Geometry check sheet. Reference: the model listing, model coordinates, mm. Round coordinates to 2 decimals unless told otherwise and drop trailing zeros. Loops run counter-clockwise (first coordinate to the right, second up) from the corner with the lowest first, then second, coordinate; pieces in that order, holes last. Notation, with made-up numbers: (-17.75, 70) -> (38.25, 70) arc R6 ccw to (38.25, 77) -> close; hole circle Ø5 at (51.5, 29). An arc over 180 degrees is marked (long way). Use one line per item in the form item = value.
from build123d import *
from OCP.BRepFilletAPI import BRepFilletAPI_MakeChamfer

# Parameters (mm, degrees)
SKETCH_1_W          = 33.5
SKETCH_1_H          = 32
SKETCH_1_R          = 1
SKETCH_1_W_2        = 23.5
SKETCH_1_H_2        = 24.25
EXTRUDE_1_DEPTH     = 2
SKETCH_2_W          = 12
SKETCH_2_H          = 12
SKETCH_2_R          = 4
EXTRUDE_2_DEPTH     = 2.2
EXTRUDE_3_DEPTH     = 12
EXTRUDE_4_DEPTH     = 12
SKETCH_5_W          = 33.5
SKETCH_5_H          = 2
EXTRUDE_5_DEPTH     = 14
SKETCH_7_W          = 2
SKETCH_7_H          = 32
EXTRUDE_6_DEPTH     = 16
SKETCH_9_R          = 3.625
CUT_EXTRUDE_1_DEPTH = 1
SKETCH_10_R         = 2.25
CUT_EXTRUDE_2_DEPTH = 1
EXTRUDE_START       = -2
SKETCH_11_R         = 5
SKETCH_11_R_2       = 3.625
EXTRUDE_7_DEPTH     = 2
FILLET_1_R          = 1
SKETCH_12_R         = 3
SKETCH_12_R_2       = 1.5
EXTRUDE_8_DEPTH     = 2
FILLET_2_R          = 1
CUT_EXTRUDE_START   = 2
SKETCH_13_R         = 1.5
CUT_EXTRUDE_3_DEPTH = 2
SKETCH_19_W         = 3.200973594
SKETCH_19_H         = 7
CUT_EXTRUDE_7_DEPTH = 10
CUT_EXTRUDE_8_DEPTH = 42
SKETCH_22_R         = 0.75
CUT_EXTRUDE_9_DEPTH = 5
CHAMFER_1_SIZE      = 1
CHAMFER_1_SIZE2     = 2


with BuildPart() as part:
    # Sketch 1 → Extrude 1 (new body)
    with BuildSketch(Plane.XY):
        with Locations((-5.75, -6.125)):
            Rectangle(SKETCH_1_W, SKETCH_1_H)
        with Locations((-20, 0)):
            Circle(SKETCH_1_R, mode=Mode.SUBTRACT)
        with Locations(Location((8.5, 0, 0), (0, 0, 180))):
            Circle(SKETCH_1_R, mode=Mode.SUBTRACT)
        with Locations(Location((-20, -12.25, 0), (0, 0, 180))):
            Circle(SKETCH_1_R, mode=Mode.SUBTRACT)
        with Locations((8.5, -12.25)):
            Circle(SKETCH_1_R, mode=Mode.SUBTRACT)
        with Locations((-5.75, -6.125)):
            Rectangle(SKETCH_1_W_2, SKETCH_1_H_2, mode=Mode.SUBTRACT)
    extrude(amount=EXTRUDE_1_DEPTH)



with BuildPart() as body_2:
    # Sketch 2 → Extrude 2 (new body)
    with BuildSketch(Plane.XY.offset(9)):
        with Locations((0, -12.25)):
            Rectangle(SKETCH_2_W, SKETCH_2_H)
        with Locations((0, -12.25)):
            Circle(SKETCH_2_R, mode=Mode.SUBTRACT)
    extrude(amount=-EXTRUDE_2_DEPTH)


with BuildPart() as part_1:
    add(part.part)

    add(body_2.part)  # Extrude 3 merges body 2
    # Sketch 3 → Extrude 3 (add)
    with BuildSketch(Plane.ZY.offset(6)):
        Polygon((9, -18.25), (2, -18.25), (2, -22.125), (9, -20.25), align=None)
    extrude(amount=-EXTRUDE_3_DEPTH)

    # Sketch 4 → Extrude 4 (add)
    with BuildSketch(Plane.ZY.offset(6)):
        Polygon((6.8, -6.25), (9, -6.25), (9, 9.5), (2, 9.5), (2, 6), (6.8, 6), align=None)
    extrude(amount=-EXTRUDE_4_DEPTH)

    # Sketch 5 → Extrude 5 (add)
    with BuildSketch(Plane(origin=(0, 0, 0), x_dir=(-1, 0, 0), z_dir=(0, 0, -1))):
        with Locations((5.75, 8.875)):
            Rectangle(SKETCH_5_W, SKETCH_5_H)
        with Locations((5.75, -21.125)):
            Rectangle(SKETCH_5_W, SKETCH_5_H)
    extrude(amount=EXTRUDE_5_DEPTH)

    # Sketch 7 → Extrude 6 (add)
    with BuildSketch(Plane.XY.offset(2)):
        with Locations((-23.5, -6.125)):
            Rectangle(SKETCH_7_W, SKETCH_7_H)
        with Locations((12, -6.125)):
            Rectangle(SKETCH_7_W, SKETCH_7_H)
    extrude(amount=-EXTRUDE_6_DEPTH)

    # Sketch 9 → Cut-Extrude 1 (cut)
    with BuildSketch(Plane(origin=(-24.5, 0, 0), x_dir=(0, 0, -1), z_dir=(1, 0, 0))):
        with Locations(Location((8, -12.25, 0), (0, 0, 90))):
            Circle(SKETCH_9_R)
    extrude(amount=CUT_EXTRUDE_1_DEPTH, mode=Mode.SUBTRACT)

    # Sketch 10 → Cut-Extrude 2 (cut)
    with BuildSketch(Plane.ZY.offset(23.5)):
        with Locations(Location((-8, -12.25, 0), (0, 0, 270))):
            Circle(SKETCH_10_R)
    extrude(amount=-CUT_EXTRUDE_2_DEPTH, mode=Mode.SUBTRACT)

    # Sketch 11 → Extrude 7 (add)
    with BuildSketch(Plane(origin=(-24.5, 0, 0), x_dir=(0, 0, -1), z_dir=(1, 0, 0)).offset(EXTRUDE_START)):
        with Locations(Location((8, -12.25, 0), (0, 0, 90))):
            Circle(SKETCH_11_R)
        with Locations(Location((8, -12.25, 0), (0, 0, 90))):
            Circle(SKETCH_11_R_2, mode=Mode.SUBTRACT)
    extrude(amount=EXTRUDE_7_DEPTH)

    # Fillet 1
    fillet_1_edges = [part_1.edges().sort_by_distance(p)[0] for p in [
        (-24.5, -17.25, -8),
    ]]
    fillet(fillet_1_edges, radius=FILLET_1_R - 0.0001)  # a hair under: the kernel refuses the full size

    # Sketch 12 → Extrude 8 (add)
    with BuildSketch(Plane.ZY.offset(-13)):
        with Locations(Location((-8, -12.25, 0), (0, 0, 270))):
            Circle(SKETCH_12_R)
        with Locations(Location((-8, -12.25, 0), (0, 0, 270))):
            Circle(SKETCH_12_R_2, mode=Mode.SUBTRACT)
    extrude(amount=-EXTRUDE_8_DEPTH)

    # Fillet 2
    fillet_2_edges = [part_1.edges().sort_by_distance(p)[0] for p in [
        (13, -9.25, -8),
    ]]
    fillet(fillet_2_edges, radius=FILLET_2_R)

    # Sketch 13 → Cut-Extrude 3 (cut)
    with BuildSketch(Plane.ZY.offset(-13).offset(CUT_EXTRUDE_START)):
        with Locations(Location((-8, -12.25, 0), (0, 0, 270))):
            Circle(SKETCH_13_R)
    extrude(amount=-CUT_EXTRUDE_3_DEPTH, mode=Mode.SUBTRACT)

    # Sketch 19 → Cut-Extrude 7 (cut)
    with BuildSketch(Plane(origin=(0, 9.5, 0), x_dir=(1, 0, 0), z_dir=(0, 1, 0))):
        with Locations((0, -5.5)):
            Rectangle(SKETCH_19_W, SKETCH_19_H)
    extrude(amount=-CUT_EXTRUDE_7_DEPTH, mode=Mode.SUBTRACT)

    # Sketch 20 → Cut-Extrude 8 (cut)
    with BuildSketch(Plane(origin=(0, 9.875, 0), x_dir=(1, 0, 0), z_dir=(0, 1, 0))):
        with BuildLine():
            Line((-7.25, 10.5), (-7.25, 1.5))
            ThreePointArc((-7.25, 1.5), (-7.542893219, 0.792893219), (-8.25, 0.5))
            Line((-8.25, 0.5), (-9.25, 0.5))
            ThreePointArc((-9.25, 0.5), (-9.957106781, 0.792893219), (-10.25, 1.5))
            Line((-10.25, 1.5), (-10.25, 10.5))
            ThreePointArc((-10.25, 10.5), (-9.957106781, 11.207106781), (-9.25, 11.5))
            Line((-9.25, 11.5), (-8.25, 11.5))
            ThreePointArc((-8.25, 11.5), (-7.542893219, 11.207106781), (-7.25, 10.5))
        make_face()
        with BuildLine():
            Line((7.75, 10.5), (7.75, 1.5))
            ThreePointArc((7.75, 1.5), (8.042893219, 0.792893219), (8.75, 0.5))
            Line((8.75, 0.5), (9.75, 0.5))
            ThreePointArc((9.75, 0.5), (10.457106781, 0.792893219), (10.75, 1.5))
            Line((10.75, 1.5), (10.75, 10.5))
            ThreePointArc((10.75, 10.5), (10.457106781, 11.207106781), (9.75, 11.5))
            Line((9.75, 11.5), (8.75, 11.5))
            ThreePointArc((8.75, 11.5), (8.042893219, 11.207106781), (7.75, 10.5))
        make_face()
        with BuildLine():
            Line((-15.25, 11.5), (-14.25, 11.5))
            ThreePointArc((-14.25, 11.5), (-13.542893219, 11.207106781), (-13.25, 10.5))
            Line((-13.25, 10.5), (-13.25, 1.5))
            ThreePointArc((-13.25, 1.5), (-13.542893219, 0.792893219), (-14.25, 0.5))
            Line((-14.25, 0.5), (-15.25, 0.5))
            ThreePointArc((-15.25, 0.5), (-15.957106781, 0.792893219), (-16.25, 1.5))
            Line((-16.25, 1.5), (-16.25, 10.5))
            ThreePointArc((-16.25, 10.5), (-15.957106781, 11.207106781), (-15.25, 11.5))
        make_face()
        with BuildLine():
            Line((-21.25, 11.5), (-20.25, 11.5))
            ThreePointArc((-20.25, 11.5), (-19.542893219, 11.207106781), (-19.25, 10.5))
            Line((-19.25, 10.5), (-19.25, 1.5))
            ThreePointArc((-19.25, 1.5), (-19.542893219, 0.792893219), (-20.25, 0.5))
            Line((-20.25, 0.5), (-21.25, 0.5))
            ThreePointArc((-21.25, 0.5), (-21.957106781, 0.792893219), (-22.25, 1.5))
            Line((-22.25, 1.5), (-22.25, 10.5))
            ThreePointArc((-22.25, 10.5), (-21.957106781, 11.207106781), (-21.25, 11.5))
        make_face()
        with BuildLine():
            Line((1.75, 10.5), (1.75, 1.5))
            ThreePointArc((1.75, 1.5), (2.042893219, 0.792893219), (2.75, 0.5))
            Line((2.75, 0.5), (3.75, 0.5))
            ThreePointArc((3.75, 0.5), (4.457106781, 0.792893219), (4.75, 1.5))
            Line((4.75, 1.5), (4.75, 10.5))
            ThreePointArc((4.75, 10.5), (4.457106781, 11.207106781), (3.75, 11.5))
            Line((3.75, 11.5), (2.75, 11.5))
            ThreePointArc((2.75, 11.5), (2.042893219, 11.207106781), (1.75, 10.5))
        make_face()
        with BuildLine():
            Line((-2.25, 11.5), (-3.25, 11.5))
            ThreePointArc((-3.25, 11.5), (-3.957106781, 11.207106781), (-4.25, 10.5))
            Line((-4.25, 10.5), (-4.25, 1.5))
            ThreePointArc((-4.25, 1.5), (-3.957106781, 0.792893219), (-3.25, 0.5))
            Line((-3.25, 0.5), (-2.25, 0.5))
            ThreePointArc((-2.25, 0.5), (-1.542893219, 0.792893219), (-1.25, 1.5))
            Line((-1.25, 1.5), (-1.25, 10.5))
            ThreePointArc((-1.25, 10.5), (-1.542893219, 11.207106781), (-2.25, 11.5))
        make_face()
    extrude(amount=-CUT_EXTRUDE_8_DEPTH, mode=Mode.SUBTRACT)

    # Sketch 22 → Cut-Extrude 9 (cut)
    with BuildSketch(Plane(origin=(0, 9.5, 0), x_dir=(1, 0, 0), z_dir=(0, 1, 0))):
        with Locations(Location((3.8, -4.8, 0), (0, 0, 270))):
            Circle(SKETCH_22_R)
        with Locations((-3.8, -4.8)):
            Circle(SKETCH_22_R)
    extrude(amount=-CUT_EXTRUDE_9_DEPTH, mode=Mode.SUBTRACT)

    # Chamfer 1: one chamfer whose edges measure the first distance from different faces: ONE call of the kernel's chamfer builder (chamfer() names one face for all edges)
    chamfer_1_edges_1 = [part_1.edges().sort_by_distance(p)[0] for p in [
        (-3.800243398, 9.5, 9),
    ]]
    chamfer_1_side_1 = [part_1.faces().sort_by_distance(p)[0] for p in [
        (-5.917322484, 9.5, 5.5),
    ]]
    chamfer_1_edges_2 = [part_1.edges().sort_by_distance(p)[0] for p in [
        (3.800243398, 9.5, 9),
    ]]
    chamfer_1_side_2 = [part_1.faces().sort_by_distance(p)[0] for p in [
        (1.683164313, 9.5, 5.5),
    ]]
    chamfer_1 = BRepFilletAPI_MakeChamfer(part_1.part.solid().wrapped)
    for e in chamfer_1_edges_1:
        chamfer_1.Add(CHAMFER_1_SIZE, CHAMFER_1_SIZE2, e.wrapped, chamfer_1_side_1[0].wrapped)  # the first distance lies on this face
    for e in chamfer_1_edges_2:
        chamfer_1.Add(CHAMFER_1_SIZE, CHAMFER_1_SIZE2, e.wrapped, chamfer_1_side_2[0].wrapped)  # the first distance lies on this face
    add(Compound.cast(chamfer_1.Shape()), mode=Mode.REPLACE)


solid = part_1.part
1. Material ranges on line 1 along X through (y, z) = (7, 4.8); line 2 along Y through (x, z) = (-20, 0.8) (3 decimals); line 3 along X through (y, z) = (-16.5, 0.5), recorded low to high.
Return value:
line_1 = -6 to -4.55, -3.05 to -1.6, 1.6 to 3.05, 4.55 to 6
line_2 = -22.125 to -13.25, -11.25 to -1, 1 to 9.875
line_3 = -24.5 to -17.5, 6 to 13
2. Section check D-D (y = -12.25). Count the separate pieces of the cut face and the enclosed holes in it, then the cut area to 3 significant figures.
Return value:
separate_pieces = 8
enclosed_holes = 0
area = 79.4 mm2
3. Gauge pin test, flat ends, axial feed: pin 1 (12 mm diameter, centred on x = -15, z = -2.5, fed in from +Y) (3 decimals); pin 2 (4 mm diameter, centred on y = -2, z = -4.5, fed in from +X); pin 3 (3 mm diameter, centred on y = 4.5, z = -2, fed in from -X); pin 4 (0.5 mm diameter, centred on x = -8.5, y = -21, fed in from +Z). Record the tip position at first contact, or that the pin passes through.
Return value:
pin_1 = 9.875
pin_2 = 13
pin_3 = -24.5
pin_4 = 2
4. Section check C-C (x = 7). Record the boundary of the cut face in (y, z) (3 decimals), then the cut area to 3 significant figures.
Return value:
outline = (-22.125, -14) -> (-20.125, -14) -> (-20.125, 0) -> (7.875, 0) -> (7.875, -14) -> (9.875, -14) -> (9.875, 2) -> (-22.125, 2) -> close
area = 120 mm2
5. Section check B-B (y = 0). Record the boundary of the cut face in (x, z).
Return value:
outline = (-24.5, -14) -> (-22.5, -14) -> (-22.5, 0) -> (-21, 0) -> (-21, 2) -> (-24.5, 2) -> close; (-19, 0) -> (-17.5, 0) -> (-17.5, 2) -> (-19, 2) -> close; (-6, 6.8) -> (-1.6, 6.8) -> (-1.6, 9) -> (-6, 9) -> close; (1.6, 6.8) -> (6, 6.8) -> (6, 9) -> (1.6, 9) -> close; (6, 0) -> (7.5, 0) -> (7.5, 2) -> (6, 2) -> close; (9.5, 0) -> (11, 0) -> (11, -14) -> (13, -14) -> (13, 2) -> (9.5, 2) -> close
6. Section check A-A (z = 1). Record the boundary of the cut face in (x, y) (3 decimals), then the cut area to 3 significant figures.
Return value:
outline = (-24.5, -22.125) -> (13, -22.125) -> (13, 9.875) -> (-24.5, 9.875) -> close; hole circle Ø2 at (-20, -12.25); hole circle Ø2 at (-20, 0); hole (-17.5, -18.25) -> (6, -18.25) -> (6, 6) -> (-17.5, 6) -> close; hole circle Ø2 at (8.5, -12.25); hole circle Ø2 at (8.5, 0)
area = 618 mm2
7. Mould release check, pull along Y, two halves, no side actions. Record for faces 1 (the cylindrical face through (4.449, 8.889, -0.785)), 2 (the cylindrical face through (-26.01, -7.48, -6.5)), 3 (the flat face through (11, -6, -7)): released by +Y, released by -Y, zero draft, split by the parting line, or undercut.
Return value:
face_1 = zero draft
face_2 = split by the parting line
face_3 = undercut
